Build history of the part. All positions in model axes, mm. A direction names the side the tool comes from. Give positions to 0.01 mm unless a question says otherwise; leave off trailing zeros. Loops run counter-clockwise (first coordinate to the right, second up) from the corner with the lowest first, then second, coordinate; pieces in that order, holes last. Notation, with made-up numbers: (-39.75, 83) -> (17.25, 83) arc R18 cw to (17.25, 107) -> close; hole circle Ø4 at (-2, 50). An arc over 180 degrees is marked (long way). Answer as a JSON object with one key per item and string values. Group by question number.
from build123d import *

# Parameters (mm, degrees)
SKETCH_R        = 23.948567
PAD_DEPTH       = 20
SKETCH001_W     = 28.280895
SKETCH001_H     = 10.191083
PAD001_DEPTH    = 20.5
PAD002_DEPTH    = 1
PAD003_DEPTH    = 10
FILLET_R        = 1
FILLET001_R     = 1
SKETCH005_W     = 23.089169
SKETCH005_H     = 7.165605
POCKET_DEPTH    = 72.73646
SKETCH006_R     = 22.653648
POCKET001_DEPTH = 20.001
POCKET002_DEPTH = 5


with BuildPart() as part:
    # Sketch → Pad (new body)
    with BuildSketch(Plane.XY):
        Circle(SKETCH_R)
    extrude(amount=PAD_DEPTH)

    # Sketch001 → Pad001 (join, symmetric)
    with BuildSketch(Plane.XZ):
        with Locations((-24.474199, 10.350326)):
            Rectangle(SKETCH001_W, SKETCH001_H)
    extrude(amount=PAD001_DEPTH, both=True)

    # Sketch002 (on Face2 of Pad001) → Pad002 (join)
    with BuildSketch(Plane(origin=(0, 0, 0), x_dir=(1, 0, 0), z_dir=(0, 0, -1))):
        with BuildLine():
            ThreePointArc((-15.78, -49.794891), (52.235424, 0), (-15.78, 49.794891))
            Line((-15.78, 49.794891), (-15.78, -49.794891))
        make_face()
    extrude(amount=-PAD002_DEPTH)

    # Sketch004 (on Face2 of Pad001) → Pad003 (join)
    with BuildSketch(Plane(origin=(0, 0, 1), x_dir=(1, 0, 0), z_dir=(0, 0, -1))):
        with BuildLine():
            ThreePointArc((-15.78, -49.794928), (52.23546, 0), (-15.78, 49.794928))
            Line((-15.78, 49.794928), (-15.78, 47.444616))
            ThreePointArc((-15.78, -47.444616), (50, 0), (-15.78, 47.444616))
            Line((-15.78, -47.444616), (-15.78, -49.794928))
        make_face()
    extrude(amount=-PAD003_DEPTH)

    # Fillet
    fillet_edges = [part.edges().sort_by_distance(p)[0] for p in [
        (50, 0, 1),
    ]]
    fillet(fillet_edges, radius=FILLET_R)

    # Fillet001
    fillet001_edges = [part.edges().sort_by_distance(p)[0] for p in [
        (52.23546, 0, 11),
        (-15.78, -48.619772, 11),
        (50, 0, 11),
        (-15.78, 48.619772, 11),
    ]]
    fillet(fillet001_edges, radius=FILLET001_R)

    # Sketch005 (on Face15 of Fillet001) → Pocket (cut, through all)
    with BuildSketch(Plane.XZ.offset(20.5)):
        with Locations((-25.879338, 10.514653)):
            Rectangle(SKETCH005_W, SKETCH005_H)
    extrude(amount=-POCKET_DEPTH, mode=Mode.SUBTRACT)

    # Sketch006 (on Face16 of Pocket) → Pocket001 (cut, through all)
    with BuildSketch(Plane.XY.offset(20)):
        Circle(SKETCH006_R)
    extrude(amount=-POCKET001_DEPTH, mode=Mode.SUBTRACT)

    # Sketch007 (on Face6 of Pocket001) → Pocket002 (cut)
    with BuildSketch(Plane.XY.offset(1)):
        with BuildLine():
            ThreePointArc((0, 40.554842), (-5.38709, 35.167753), (0, 29.780663))
            ThreePointArc((26.742534, 13.104381), (15.758026, 25.269993), (0, 29.780663))
            ThreePointArc((26.742534, 13.104381), (33.950529, 10.637346), (36.417565, 17.845341))
            ThreePointArc((36.417565, 17.845341), (21.459033, 34.412281), (0, 40.554842))
        make_face()
        with BuildLine():
            ThreePointArc((0, -29.780663), (-5.38709, -35.167753), (0, -40.554842))
            ThreePointArc((0, -40.554842), (21.459033, -34.412281), (36.417565, -17.845341))
            ThreePointArc((36.417565, -17.845341), (33.950529, -10.637346), (26.742534, -13.104381))
            ThreePointArc((0, -29.780663), (15.758026, -25.269993), (26.742534, -13.104381))
        make_face()
    extrude(amount=-POCKET002_DEPTH, mode=Mode.SUBTRACT)


solid = part.part
(1) Saw through at A-A on z = 3.25. List the corners of the cut face in (x, y), plus the area to 3 significant figures.
(2) 3-axis set-ups, long thin cutter, end or side, ignore diameter. For faces 1 (the flat face through (-24.6, 20.5, 6.6)), 2 (the cylindrical face through (15.95, 25.15, 0.51)), 3 (the flat face through (-14.335, 19, 10)), 4 (the flat face through (-29, 0, 14.097)), 5 (the cylindrical face through (49.982, 1.324, 5.944)): which of +Z, -Z, +X, -X, +Y, -Y reach the whole face in a straight line?
(3) Saw through at B-B on x = -20.5. List the corners of the cut face in (y, z), plus the area to 3 significant figures.
(4) Pin check, flat tips, straight feed: pin 1 (6 mm diameter, centred on x = 21, z = 8, fed in from -Y); pin 2 (7.5 mm diameter, centred on y = 36, z = 4.5, fed in from -X); pin 3 (11 mm diameter, centred on x = -25.5, z = 11, fed in from -Y); pin 4 (7 mm diameter, centred on x = -21, y = -5.5, fed in from +Z). Stop position of each tip, or through.
(5) Probe line 1 along X through (y, z) = (0, 6.25); line 2 along Y through (x, z) = (0, 5.75); line 3 along Y through (x, z) = (0, 13.5). List the from-to ranges inside material, lowest first. Write a range as [from, to].
(6) Pull direction Y, two halves, no side cores. Call faces 6 (the cylindrical face through (52.217, 1.373, 0.493)), 7 (the cylindrical face through (-5.386, -35.049, 0.507)), 8 (the flat face through (-37.424, 0, 10)): pulls with the +Y half, pulls with the -Y half, needs draft (parallel to the pull), parting line crosses it, or undercut.
(7) Saw through at C-C on z = 8.25. List the corners of the cut face in (x, y).
Calculated:
{
 "1": {"outline": "circle Ø47.9 at (0, 0); (-15.78, -49.79) arc R52.24 ccw (long way) to (-15.78, 49.79) -> (-15.78, 47.44) arc R50 cw (long way) to (-15.78, -47.44) -> close; hole circle Ø45.31 at (0, 0)", "area": "620 mm^2"},
 "2": {"face 1": "+Z, -X", "face 2": "+Z, -Z", "face 3": "+Y", "face 4": "+Y, -Y", "face 5": "+Z"},
 "3": {"outline": "(-20.5, 5.25) -> (-12.38, 5.25) -> (-12.38, 0) -> (-9.64, 0) -> (-9.64, 6.93) -> (-20.5, 6.93) -> close; (-20.5, 14.1) -> (-9.64, 14.1) -> (-9.64, 20) -> (-12.38, 20) -> (-12.38, 15.45) -> (-20.5, 15.45) -> close; (9.64, 0) -> (12.38, 0) -> (12.38, 5.25) -> (20.5, 5.25) -> (20.5, 6.93) -> (9.64, 6.93) -> close; (9.64, 14.1) -> (20.5, 14.1) -> (20.5, 15.45) -> (12.38, 15.45) -> (12.38, 20) -> (9.64, 20) -> close", "area": "119 mm^2"},
 "4": {"pin 1": "stops at y = -49.04", "pin 2": "stops at x = -15.78", "pin 3": "stops at y = -20.5", "pin 4": "stops at z = 20"},
 "5": {"line 1": "x = [-38.61, -22.65], [22.65, 23.95], [50, 52.24]", "line 2": "y = [-52.24, -50], [-23.95, -22.65], [22.65, 23.95], [50, 52.24]", "line 3": "y = [-23.95, -22.65], [22.65, 23.95]"},
 "6": {"face 6": "parting line crosses it", "face 7": "undercut", "face 8": "needs draft"},
 "7": {"outline": "(-38.61, -20.5) -> (-37.42, -20.5) -> (-37.42, 20.5) -> (-38.61, 20.5) -> close; (-15.78, -49.79) arc R52.24 ccw (long way) to (-14.33, 50.23) -> (-14.33, 47.9) arc R50 cw (long way) to (-15.78, -47.44) -> close; (-14.33, -20.5) -> (-12.38, -20.5) arc R23.95 ccw (long way) to (-12.38, 20.5) -> (-14.33, 20.5) -> (-14.33, 17.54) arc R22.65 cw (long way) to (-14.33, -17.54) -> close"}
}
